from build123d import *

# Parameters (mm, degrees)
CYLINDER_R             = 4.2
CYLINDER_DEPTH         = 46
CYLINDER001_R          = 2.1
CYLINDER001_DEPTH      = 46
SKETCH001_W            = 2
SKETCH001_H            = 14
PAD001_DEPTH           = 46
CYLINDER003_R          = 2.95
CYLINDER003_DEPTH      = 4
CYLINDER002_R          = 1.9
CYLINDER002_DEPTH      = 10
PRISM_DEPTH            = 3
FUSION_ROLL_ANGLE      = -90.000052
FUSION_PITCH_ANGLE     = -59.999967
FUSION_PLACEMENT_ANGLE = 90.000052
PAD004_DEPTH           = 10
PAD006_DEPTH           = 15
PAD_DEPTH              = 44
PAD005_DEPTH           = 34


with BuildPart() as rod_cut:
    # Cylinder → Cylinder (new body)
    with BuildSketch(Plane(origin=(-30, 0, -1), x_dir=(1, 0, 0), z_dir=(0, 0, 1))):
        Circle(CYLINDER_R)
    extrude(amount=CYLINDER_DEPTH)


with BuildPart() as top_screw_cut:
    # Cylinder001 → Cylinder001 (new body)
    with BuildSketch(Plane(origin=(-30, 12, -1), x_dir=(1, 0, 0), z_dir=(0, 0, 1))):
        Circle(CYLINDER001_R)
    extrude(amount=CYLINDER001_DEPTH)


with BuildPart() as clamps_relief_cut:
    # Sketch001 → Pad001 (new body)
    with BuildSketch(Plane.XY.offset(-1)):
        with Locations((-30, -7)):
            Rectangle(SKETCH001_W, SKETCH001_H)
    extrude(amount=PAD001_DEPTH)


with BuildPart() as cylinder001:
    # Cylinder003 → Cylinder003 (new body)
    with BuildSketch(Plane.XY.offset(10)):
        Circle(CYLINDER003_R)
    extrude(amount=CYLINDER003_DEPTH)


with BuildPart() as cylinder:
    # Cylinder002 → Cylinder002 (new body)
    with BuildSketch(Plane.XY):
        Circle(CYLINDER002_R)
    extrude(amount=CYLINDER002_DEPTH)


with BuildPart() as fusion:
    # Prism → Prism (new body)
    with BuildSketch(Plane.XY.offset(-1)):
        Polygon((3.45, 0), (1.725, 2.987788), (-1.725, 2.987788), (-3.45, 0), (-1.725, -2.987788), (1.725, -2.987788), align=None)
    extrude(amount=PRISM_DEPTH)

    # Fusion: union Cylinder001, Cylinder
    add(cylinder001.part)
    add(cylinder.part)


with BuildPart() as fusion_1:
    # Fusion roll: moved
    add(fusion.part.rotate(Axis((0, 0, 0), (1, 0, 0)), FUSION_ROLL_ANGLE))


with BuildPart() as fusion_2:
    # Fusion pitch: moved
    add(fusion_1.part.rotate(Axis((0, 0, 0), (0, 1, 0)), FUSION_PITCH_ANGLE))


with BuildPart() as fusion_3:
    # Fusion placement: moved
    add(fusion_2.part.moved(Location((-24, -7.5, 7))).rotate(Axis((-24, -7.5, 7), (0, 0, 1)), FUSION_PLACEMENT_ANGLE))


with BuildPart() as clone_of_fusion:
    # Clone base: copy of Fusion
    add(fusion_3.part)


with BuildPart() as clone_of_fusion_1:
    # Clone placement: moved
    add(clone_of_fusion.part.moved(Location((0, 0, 14))))


with BuildPart() as fusion006005:
    # Clone001 base: copy of Fusion
    add(fusion_3.part)


with BuildPart() as fusion006005_1:
    # Clone001 placement: moved
    add(fusion006005.part.moved(Location((0, 0, 28))))

    # Fusion006005: union Clone of Fusion, Fusion
    add(clone_of_fusion_1.part)
    add(fusion_3.part)


with BuildPart() as fusion006006:
    # Clone002 base: copy of Top_screw_cut
    add(top_screw_cut.part)


with BuildPart() as fusion006006_1:
    # Clone002 placement: moved
    add(fusion006006.part.moved(Location((0, 35, 0))))

    # Fusion006006: union Rod_cut, Top_screw_cut, Clamps_Relief_cut, Fusion006005
    add(rod_cut.part)
    add(top_screw_cut.part)
    add(clamps_relief_cut.part)
    add(fusion006005_1.part)


with BuildPart() as fusion006008:
    # Sketch004 → Pad004 (new body)
    with BuildSketch(Plane.XZ.offset(-4)):
        with BuildLine():
            ThreePointArc((-8.485281, 30.485281), (-2e-06, 10), (8.485284, 30.485278))
            Line((0, 38.970563), (8.485284, 30.485278))
            Line((-8.485281, 30.485281), (0, 38.970563))
        make_face()
        Polygon((-18.879751, 38.475588), (-16.475588, 40.879751), (-10.111627, 34.51579), (-12.51579, 32.111627), align=None)
        Polygon((-18.879751, 5.524412), (-12.51579, 11.888373), (-10.111627, 9.48421), (-16.475588, 3.120249), align=None)
    extrude(amount=-PAD004_DEPTH)

    # Fusion006008: union Fusion006006
    add(fusion006006_1.part)


with BuildPart() as pad006:
    # Sketch007 → Pad006 (new body)
    with BuildSketch(Plane.YZ.offset(-22)):
        Polygon((17, 35), (42, 10), (58.138325, 10), (58.138325, 51.535988), (17, 51.535988), align=None)
    extrude(amount=-PAD006_DEPTH)


with BuildPart() as idler_half_raw:
    # Sketch → Pad (new body)
    with BuildSketch(Plane.XY):
        with BuildLine():
            ThreePointArc((-24, 10), (-30, 16), (-36, 10))
            Line((-36, -12), (-36, 10))
            Line((-24, -12), (-36, -12))
            Line((-24, 5), (-24, -12))
            Line((0, 5), (-24, 5))
            Line((0, 10), (0, 5))
            Line((-24, 10), (0, 10))
        make_face()
    extrude(amount=PAD_DEPTH)


with BuildPart() as cut001:
    # Sketch005 → Pad005 (new body)
    with BuildSketch(Plane.XY):
        with BuildLine():
            Line((-27.5, 15), (-32.5, 15))
            Line((-32.5, 15), (-32.5, 42.669873))
            ThreePointArc((-27.5, 42.669873), (-30, 52), (-32.5, 42.669873))
            Line((-27.5, 42.669873), (-27.5, 15))
        make_face()
    extrude(amount=PAD005_DEPTH)

    # Fusion006007: union Idler_Half_Raw
    add(idler_half_raw.part)

    # Cut: cut Pad006
    add(pad006.part, mode=Mode.SUBTRACT)

    # Cut001: cut Fusion006008
    add(fusion006008.part, mode=Mode.SUBTRACT)


with BuildPart() as fusion006009:
    # Part__Mirroring: instance of Cut001
    add(cut001.part.mirror(Plane(origin=(0, 0, 0), x_dir=(0, -1, 0), z_dir=(1, 0, 0))))

    # Fusion006009: union Cut001
    add(cut001.part)


solid = fusion006009.part
Check sheet for the modelled part. Datum: model origin and axes. Units: mm. A direction names the side the tool comes from. Give positions to 0.01 mm unless a question says otherwise; leave off trailing zeros. Write each loop counter-clockwise with the first axis right and the second up, starting at its lowest first coordinate (ties: lowest second). Pieces come first, ordered by that corner, then holes. Notation, with made-up numbers: (8.5, 82.25) -> (22.5, 82.25) arc R9 ccw to (22.5, 98.25) -> close; hole circle Ø1 at (1, -22.75). An arc over 180 degrees is marked (long way). Use one line per item in the form item = value. Start each with the question number.
1. Section check A-A (y = 47). Record the cut outline in (x, z).
2. Mould release check, pull along Y, two halves, no side actions. Record for faces 5 (the cylindrical face through (-27.479, -7.088, 19.145)), 6 (the flat face through (-26, -12, 22)), 7 (the flat face through (11.3, 7.46, 33.33)): pulls with the +Y half, pulls with the -Y half, needs draft (parallel to the pull), parting line crosses it, or undercut.
3. Access from +Z, -Z, +X, -X, +Y, -Y to the whole of each face (thin tool, end or side, straight path). Record for faces 1 (the flat face through (26, -8, 9)), 2 (the flat face through (-29, -10, 22)), 3 (the flat face through (-34, -7, 9)), 4 (the flat face through (34, -7, 23)).
4. Section check B-B (z = 26). Count the separate pieces of the cut face and the enclosed holes in it, and give its area (3 significant figures).
5. Go/stop test with flat-tipped pins: P1, Ø5, axis at x = 17.5, z = 6.5, coming from the +Y side; P2, Ø3.5, axis at y = -7.5, z = 7, coming from the -X side; P3, Ø8, axis at y = 25, z = 13, coming from the -X side; P4, Ø5.5, axis at y = -7.5, z = 7, coming from the -X side. Record where each tip stops, or that it passes through.
6. Section check D-D (x = 30). Record the cut outline in (y, z).
7. Thickness scan on line 1 along X through (y, z) = (-7.5, 14.5); line 2 along Z through (x, y) = (26.8, -7.5); line 3 along X through (y, z) = (-3, 4.5). Record the ranges inside material, lowest first. Write a range as from..to.
8. Section check C-C (y = 29.5). Record the cut outline in (x, z), and give its area (3 significant figures).
Conclusion:
q1.outline = (-35, 0) -> (-32.1, 0) -> (-32.1, 10) -> (-35, 10) -> close; (-27.9, 0) -> (-25, 0) -> (-25, 10) -> (-27.9, 10) -> close; (25, 0) -> (27.9, 0) -> (27.9, 10) -> (25, 10) -> close; (32.1, 0) -> (35, 0) -> (35, 10) -> (32.1, 10) -> close
q2.face_5 = undercut
q2.face_6 = pulls with the -Y half
q2.face_7 = needs draft
q3.face_1 = none
q3.face_2 = +Z, -Z, -Y
q3.face_3 = -X
q3.face_4 = +X
q4.separate_pieces = 2
q4.enclosed_holes = 2
q4.area = 700 mm²
q5.P1 = 10
q5.P2 = through
q5.P3 = -32.5
q5.P4 = -34
q6.outline = (4.2, 0) -> (9.9, 0) -> (9.9, 44) -> (4.2, 44) -> close; (14.1, 0) -> (44.9, 0) -> (44.9, 10) -> (42, 10) -> (18, 34) -> (16, 34) -> (16, 44) -> (14.1, 44) -> close; (49.1, 0) -> (52, 0) -> (52, 10) -> (49.1, 10) -> close
q7.line_1 = -36..-31, -29..-24, 24..29, 31..36
q7.line_2 = 0..5.1, 8.9..19.1, 22.9..33.1, 36.9..44
q7.line_3 = -36..-32.94, -27.06..-24, 24..27.06, 32.94..36
q8.outline = (-32.5, 0) -> (-27.5, 0) -> (-27.5, 22.5) -> (-32.5, 22.5) -> close; (27.5, 0) -> (32.5, 0) -> (32.5, 22.5) -> (27.5, 22.5) -> close
q8.area = 225 mm²
